Can you work these out from the model? Positions are in its coordinate system, mm. Face numbers are marked on the shaded views. Give positions to 0.01 mm unless a question says otherwise; leave off trailing zeros. Write each loop counter-clockwise with the first axis right and the second up, starting at its lowest first coordinate (ties: lowest second). Pieces come first, ordered by that corner, then holes. Notation, with made-up numbers: (3, -33.75) -> (45, -33.75) arc R20 ccw to (45, -2.75) -> close; hole circle Ø1 at (32, 83.25). An arc over 180 degrees is marked (long way). One line per item, written item: value.
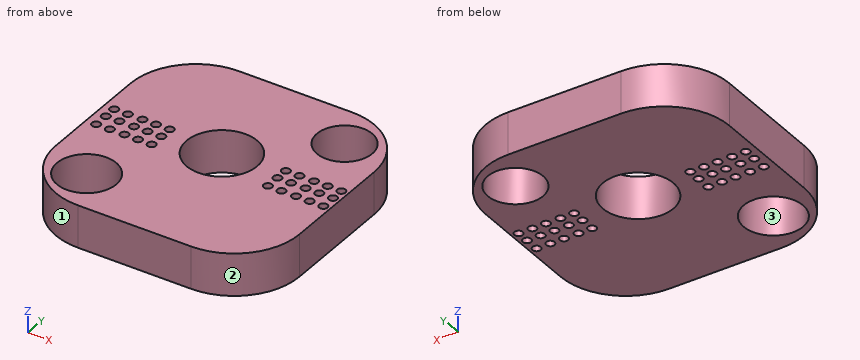
from build123d import *

# Parameters (mm, degrees)
SKETCH_R     = 25
SKETCH_R_2   = 21
SKETCH_R_3   = 19.584537
SKETCH_R_4   = 3
PAD_DEPTH    = 30
PAD001_DEPTH = 30


with BuildPart() as part:
    # Sketch → Pad (new body)
    with BuildSketch(Plane.XY):
        with BuildLine():
            Line((-35.584206, -63.111127), (44.415794, -63.111127))
            ThreePointArc((44.415794, -63.111127), (77.13309, -49.55918), (90.685038, -16.841884))
            Line((90.685038, -16.841884), (90.685038, 63.158116))
            ThreePointArc((90.685038, 63.158116), (77.13309, 95.875412), (44.415794, 109.427359))
            Line((44.415794, 109.427359), (-35.584206, 109.427359))
            ThreePointArc((-35.584206, 109.427359), (-68.301501, 95.875412), (-81.853449, 63.158116))
            Line((-81.853449, 63.158116), (-81.853449, -16.841884))
            ThreePointArc((-81.853449, -16.841884), (-68.301501, -49.55918), (-35.584206, -63.111127))
        make_face()
        with Locations((4.62833, 30.241158)):
            Circle(SKETCH_R, mode=Mode.SUBTRACT)
        with Locations((-50.106209, -31.898642)):
            Circle(SKETCH_R_2, mode=Mode.SUBTRACT)
        with Locations((59.362869, 78.858307)):
            Circle(SKETCH_R_3, mode=Mode.SUBTRACT)
        with Locations((-74.575775, 34.748711)):
            Circle(SKETCH_R_4, mode=Mode.SUBTRACT)
        with Locations((-64.916733, 34.748711)):
            Circle(SKETCH_R_4, mode=Mode.SUBTRACT)
        with Locations((-54.613762, 34.748711)):
            Circle(SKETCH_R_4, mode=Mode.SUBTRACT)
        with Locations((-44.95472, 34.748711)):
            Circle(SKETCH_R_4, mode=Mode.SUBTRACT)
        with Locations((-35.295681, 34.748711)):
            Circle(SKETCH_R_4, mode=Mode.SUBTRACT)
        with Locations((-74.575775, 25.733604)):
            Circle(SKETCH_R_4, mode=Mode.SUBTRACT)
        with Locations((-64.916733, 25.733604)):
            Circle(SKETCH_R_4, mode=Mode.SUBTRACT)
        with Locations((-54.613762, 25.733604)):
            Circle(SKETCH_R_4, mode=Mode.SUBTRACT)
        with Locations((-44.95472, 25.733604)):
            Circle(SKETCH_R_4, mode=Mode.SUBTRACT)
        with Locations((-35.295681, 25.733604)):
            Circle(SKETCH_R_4, mode=Mode.SUBTRACT)
        with Locations((-74.575775, 15.430638)):
            Circle(SKETCH_R_4, mode=Mode.SUBTRACT)
        with Locations((-64.916733, 15.430638)):
            Circle(SKETCH_R_4, mode=Mode.SUBTRACT)
        with Locations((-54.613762, 15.430638)):
            Circle(SKETCH_R_4, mode=Mode.SUBTRACT)
        with Locations((-44.95472, 15.430638)):
            Circle(SKETCH_R_4, mode=Mode.SUBTRACT)
        with Locations((-35.295681, 15.430638)):
            Circle(SKETCH_R_4, mode=Mode.SUBTRACT)
        with Locations((46.484135, 35.392643)):
            Circle(SKETCH_R_4, mode=Mode.SUBTRACT)
        with Locations((56.143177, 35.392643)):
            Circle(SKETCH_R_4, mode=Mode.SUBTRACT)
        with Locations((66.446148, 35.392643)):
            Circle(SKETCH_R_4, mode=Mode.SUBTRACT)
        with Locations((76.10519, 35.392643)):
            Circle(SKETCH_R_4, mode=Mode.SUBTRACT)
        with Locations((85.764229, 35.392643)):
            Circle(SKETCH_R_4, mode=Mode.SUBTRACT)
        with Locations((46.484135, 26.377536)):
            Circle(SKETCH_R_4, mode=Mode.SUBTRACT)
        with Locations((56.143177, 26.377536)):
            Circle(SKETCH_R_4, mode=Mode.SUBTRACT)
        with Locations((66.446148, 26.377536)):
            Circle(SKETCH_R_4, mode=Mode.SUBTRACT)
        with Locations((76.10519, 26.377536)):
            Circle(SKETCH_R_4, mode=Mode.SUBTRACT)
        with Locations((85.764229, 26.377536)):
            Circle(SKETCH_R_4, mode=Mode.SUBTRACT)
        with Locations((46.484135, 16.07457)):
            Circle(SKETCH_R_4, mode=Mode.SUBTRACT)
        with Locations((56.143177, 16.07457)):
            Circle(SKETCH_R_4, mode=Mode.SUBTRACT)
        with Locations((66.446148, 16.07457)):
            Circle(SKETCH_R_4, mode=Mode.SUBTRACT)
        with Locations((76.10519, 16.07457)):
            Circle(SKETCH_R_4, mode=Mode.SUBTRACT)
        with Locations((85.764229, 16.07457)):
            Circle(SKETCH_R_4, mode=Mode.SUBTRACT)
    extrude(amount=PAD_DEPTH)

    # Sketch → Pad001 (join)
    with BuildSketch(Plane.XY):
        with BuildLine():
            Line((-35.584206, -63.111127), (44.415794, -63.111127))
            ThreePointArc((44.415794, -63.111127), (77.13309, -49.55918), (90.685038, -16.841884))
            Line((90.685038, -16.841884), (90.685038, 63.158116))
            ThreePointArc((90.685038, 63.158116), (77.13309, 95.875412), (44.415794, 109.427359))
            Line((44.415794, 109.427359), (-35.584206, 109.427359))
            ThreePointArc((-35.584206, 109.427359), (-68.301501, 95.875412), (-81.853449, 63.158116))
            Line((-81.853449, 63.158116), (-81.853449, -16.841884))
            ThreePointArc((-81.853449, -16.841884), (-68.301501, -49.55918), (-35.584206, -63.111127))
        make_face()
        with Locations((4.62833, 30.241158)):
            Circle(SKETCH_R, mode=Mode.SUBTRACT)
        with Locations((-50.106209, -31.898642)):
            Circle(SKETCH_R_2, mode=Mode.SUBTRACT)
        with Locations((59.362869, 78.858307)):
            Circle(SKETCH_R_3, mode=Mode.SUBTRACT)
        with Locations((-74.575775, 34.748711)):
            Circle(SKETCH_R_4, mode=Mode.SUBTRACT)
        with Locations((-64.916733, 34.748711)):
            Circle(SKETCH_R_4, mode=Mode.SUBTRACT)
        with Locations((-54.613762, 34.748711)):
            Circle(SKETCH_R_4, mode=Mode.SUBTRACT)
        with Locations((-44.95472, 34.748711)):
            Circle(SKETCH_R_4, mode=Mode.SUBTRACT)
        with Locations((-35.295681, 34.748711)):
            Circle(SKETCH_R_4, mode=Mode.SUBTRACT)
        with Locations((-74.575775, 25.733604)):
            Circle(SKETCH_R_4, mode=Mode.SUBTRACT)
        with Locations((-64.916733, 25.733604)):
            Circle(SKETCH_R_4, mode=Mode.SUBTRACT)
        with Locations((-54.613762, 25.733604)):
            Circle(SKETCH_R_4, mode=Mode.SUBTRACT)
        with Locations((-44.95472, 25.733604)):
            Circle(SKETCH_R_4, mode=Mode.SUBTRACT)
        with Locations((-35.295681, 25.733604)):
            Circle(SKETCH_R_4, mode=Mode.SUBTRACT)
        with Locations((-74.575775, 15.430638)):
            Circle(SKETCH_R_4, mode=Mode.SUBTRACT)
        with Locations((-64.916733, 15.430638)):
            Circle(SKETCH_R_4, mode=Mode.SUBTRACT)
        with Locations((-54.613762, 15.430638)):
            Circle(SKETCH_R_4, mode=Mode.SUBTRACT)
        with Locations((-44.95472, 15.430638)):
            Circle(SKETCH_R_4, mode=Mode.SUBTRACT)
        with Locations((-35.295681, 15.430638)):
            Circle(SKETCH_R_4, mode=Mode.SUBTRACT)
        with Locations((46.484135, 35.392643)):
            Circle(SKETCH_R_4, mode=Mode.SUBTRACT)
        with Locations((56.143177, 35.392643)):
            Circle(SKETCH_R_4, mode=Mode.SUBTRACT)
        with Locations((66.446148, 35.392643)):
            Circle(SKETCH_R_4, mode=Mode.SUBTRACT)
        with Locations((76.10519, 35.392643)):
            Circle(SKETCH_R_4, mode=Mode.SUBTRACT)
        with Locations((85.764229, 35.392643)):
            Circle(SKETCH_R_4, mode=Mode.SUBTRACT)
        with Locations((46.484135, 26.377536)):
            Circle(SKETCH_R_4, mode=Mode.SUBTRACT)
        with Locations((56.143177, 26.377536)):
            Circle(SKETCH_R_4, mode=Mode.SUBTRACT)
        with Locations((66.446148, 26.377536)):
            Circle(SKETCH_R_4, mode=Mode.SUBTRACT)
        with Locations((76.10519, 26.377536)):
            Circle(SKETCH_R_4, mode=Mode.SUBTRACT)
        with Locations((85.764229, 26.377536)):
            Circle(SKETCH_R_4, mode=Mode.SUBTRACT)
        with Locations((46.484135, 16.07457)):
            Circle(SKETCH_R_4, mode=Mode.SUBTRACT)
        with Locations((56.143177, 16.07457)):
            Circle(SKETCH_R_4, mode=Mode.SUBTRACT)
        with Locations((66.446148, 16.07457)):
            Circle(SKETCH_R_4, mode=Mode.SUBTRACT)
        with Locations((76.10519, 16.07457)):
            Circle(SKETCH_R_4, mode=Mode.SUBTRACT)
        with Locations((85.764229, 16.07457)):
            Circle(SKETCH_R_4, mode=Mode.SUBTRACT)
    extrude(amount=PAD001_DEPTH)


solid = part.part
1) If we section it at A-A (y = 67): Write out the boundary of the cut face in (x, z), and give its area (3 significant figures).
Answer list:
outline: (-81.69, 0) -> (43.78, 0) -> (43.78, 30) -> (-81.69, 30) -> close; (74.95, 0) -> (90.53, 0) -> (90.53, 30) -> (74.95, 30) -> close
area: 4,230 mm^2
2) I need wall thicknesses on L1, parallel to Y at x = 75.5, z = 18.5; L2, parallel to Y at x = -44, z = 1.75; L3, parallel to X at y = -29, z = 24. Which ranges of each line are inside material? Lowest first, please.
Answer list:
L1: y = -51.11 to 13.14, 19.01 to 23.44, 29.32 to 32.45, 38.33 to 67.76, 89.96 to 97.43
L2: y = -62.34 to -51.99, -11.81 to 12.59, 18.27 to 22.89, 28.58 to 31.9, 37.59 to 108.66
L3: x = -80.23 to -70.91, -29.31 to 89.06
3) If we section it at C-C (z = 22): State how many separate pieces and enclosed holes the cut face has, and give its area (3 significant figures).
Answer list:
separate pieces: 1
enclosed holes: 33
area: 22,500 mm^2
4) Will these pins go through, and if not, where does the flat tip stop? pin 1 (3.5 mm diameter, centred on x = -54.61, y = 15.43, fed in from +Z); pin 2 (4 mm diameter, centred on y = 66.5, z = 7.5, fed in from -X).
Answer list:
pin 1: passes through
pin 2: stops at x = -81.83
5) If we section it at B-B (x = 4.5): Write out the boundary of the cut face in (y, z).
Answer list:
outline: (-63.11, 0) -> (5.24, 0) -> (5.24, 30) -> (-63.11, 30) -> close; (55.24, 0) -> (109.43, 0) -> (109.43, 30) -> (55.24, 30) -> close
6) We'd pull the mould along X, two halves only. Please class the marked faces 1, 2 and 3: released by +X, released by -X, zero draft, split by the parting line, or undercut.
Answer list:
face 1: released by -X
face 2: released by +X
face 3: undercut
